Input: part model. Units: mm. Frame: model coordinates. Face numbers are marked on the shaded views. A direction names the side the tool comes from. Round coordinates to 2 decimals unless told otherwise and drop trailing zeros. Loops run counter-clockwise (first coordinate to the right, second up) from the corner with the lowest first, then second, coordinate; pieces in that order, holes last.
(1) First-contact query: pin 1 Ø12 at (x, y) = (-6, 8.5) entering from -Z; pin 2 Ø1.6 at (x, z) = (22.76, -15.21) entering from -Y; pin 3 Ø6 at (x, y) = (13.5, 15) entering from -Z. Flat tips, straight axial feed; report the tip coordinate or a pass-through.
(2) Access query for the marked faces 1 and 2. Directions: +Z, -Z, +X, -X, +Y, -Y. A direction counts if a zero-diameter tool reaches every point of the face in a straight line with its end or side. Return the directions, or none.
(3) Draft query along Z for the marked faces 3, 4 and 5. Return one class per face: released by +Z, released by -Z, zero draft, split by the parting line, or undercut.
(4) Cut plane D-D, the plane x = 8. Output: boundary loops of the cut face in (y, z), and give its area (3 significant figures).
(5) Cut plane B-B, the plane x = 0. Output: boundary loops of the cut face in (y, z).
(6) Cut plane A-A, the plane z = 0. Output: boundary loops of the cut face in (x, y), and give its area (3 significant figures).
(7) Cut plane C-C, the plane y = 30.5. Output: boundary loops of the cut face in (x, z).
(8) Line query: line 1 (Y direction, x = -7, z = -26.5); line 2 (X direction, y = 30.5, z = -1.5); line 3 (X direction, y = 24, z = -11). Output: solid intervals per line, ascending.
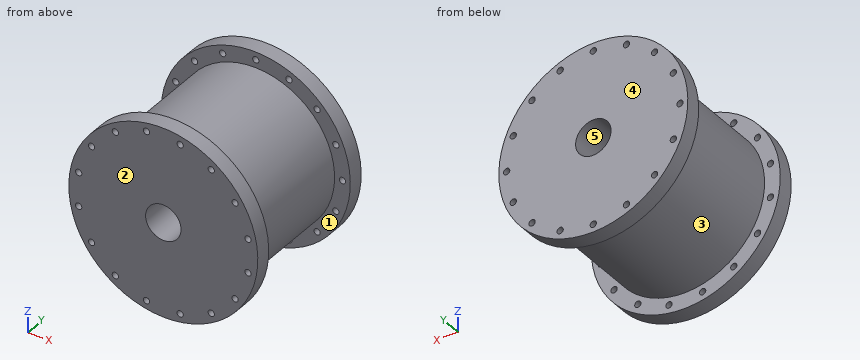
from build123d import *

# Parameters (mm, degrees)
SKETCH4_R          = 5.621513677
CUT_EXTRUDE1_DEPTH = 64.627776498
SKETCH5_R          = 1
CUT_EXTRUDE2_DEPTH = 60.991308336
CIRPATTERN2_COUNT  = 16
CUT_EXTRUDE3_REACH = 65.628
SKETCH7_R          = 1
CIRPATTERN3_COUNT  = 16


with BuildPart() as part:
    # Sketch3 → Revolve1 (revolve)
    with BuildSketch(Plane(origin=(0, 0, 0), x_dir=(0, 0, -1), z_dir=(1, 0, 0))):
        Polygon((29.972, 0), (0, 0), (0, 47.453686622), (29.972, 47.453686622), (29.972, 42.453686622), (24.993307857, 42.453686622), (24.993307857, 5), (29.972, 5), align=None)
    revolve(axis=Axis((0, 47.453686622, 0), (0, 1, 0)))

    # Sketch4 → Cut-Extrude1 (cut, through all)
    with BuildSketch(Plane(origin=(0, 47.453686622, 0), x_dir=(1, 0, 0), z_dir=(0, 1, 0))):
        with Locations(Location((0, 0, 0), (0, 0, 270))):
            Circle(SKETCH4_R)
    extrude(amount=-CUT_EXTRUDE1_DEPTH, mode=Mode.SUBTRACT)

    # Sketch5 → Cut-Extrude2 (cut, through all)
    with BuildSketch(Plane.XZ.offset(-42.453686622)):
        with Locations(Location((0, 27.482653928, 0), (0, 0, 270))):
            Circle(SKETCH5_R)
    cut_extrude2 = extrude(amount=-CUT_EXTRUDE2_DEPTH, mode=Mode.SUBTRACT)

    # CirPattern2: Cut-Extrude2 ×16 about axis
    cirpattern2_axis = Axis((0, 0, 0), (0, 1, 0))
    for i in range(1, CIRPATTERN2_COUNT):
        add(cut_extrude2.rotate(cirpattern2_axis, i * 360 / CIRPATTERN2_COUNT), mode=Mode.SUBTRACT)

    # Sketch7 → Cut-Extrude3 (cut, up to next)
    with BuildSketch(Plane.XZ, mode=Mode.PRIVATE) as cut_extrude3_sk1:
        with Locations(Location((-5.341086171, 26.85145344, 0), (0, 0, 270))):
            Circle(SKETCH7_R)
    cut_extrude3_tool1 = extrude(cut_extrude3_sk1.sketch, amount=-CUT_EXTRUDE3_REACH, mode=Mode.PRIVATE) & part.part
    cut_extrude3 = cut_extrude3_tool1.solids().sort_by_distance((-5.341086, 0, 26.851453))[0]
    add(cut_extrude3, mode=Mode.SUBTRACT)

    # CirPattern3: Cut-Extrude3 ×16 about axis
    cirpattern3_axis = Axis((0, 0, 0), (0, 1, 0))
    for i in range(1, CIRPATTERN3_COUNT):
        add(cut_extrude3.rotate(cirpattern3_axis, i * 360 / CIRPATTERN3_COUNT), mode=Mode.SUBTRACT)


solid = part.part
Reported:
1. pin 1: stops at z = -29.95
1. pin 2: stops at y = 42.45
1. pin 3: stops at z = -22.68
2. face 1: none
2. face 2: +Z, -Z, +X, -X, -Y
3. face 3: split by the parting line
3. face 4: zero draft
3. face 5: undercut
4. outline: (0, -28.88) - (5, -28.88) - (5, -23.68) - (42.45, -23.68) - (42.45, -28.88) - (47.45, -28.88) - (47.45, 28.88) - (42.45, 28.88) - (42.45, 23.68) - (5, 23.68) - (5, 28.88) - (0, 28.88) - close
4. area: 2,350 mm2
5. outline: (0, -29.97) - (5, -29.97) - (5, -24.99) - (42.45, -24.99) - (42.45, -26.48) - (47.45, -26.48) - (47.45, -5.62) - (0, -5.62) - close; (0, 5.62) - (47.45, 5.62) - (47.45, 26.48) - (42.45, 26.48) - (42.45, 24.99) - (5, 24.99) - (5, 29.97) - (0, 29.97) - close; (42.45, -29.97) - (47.45, -29.97) - (47.45, -28.48) - (42.45, -28.48) - close; (42.45, 28.48) - (47.45, 28.48) - (47.45, 29.97) - (42.45, 29.97) - close
6. outline: (-29.97, 0) - (-5.62, 0) - (-5.62, 47.45) - (-26.48, 47.45) - (-26.48, 42.45) - (-24.99, 42.45) - (-24.99, 5) - (-29.97, 5) - close; (-29.97, 42.45) - (-28.48, 42.45) - (-28.48, 47.45) - (-29.97, 47.45) - close; (5.62, 0) - (29.97, 0) - (29.97, 5) - (24.99, 5) - (24.99, 42.45) - (26.48, 42.45) - (26.48, 47.45) - (5.62, 47.45) - close; (28.48, 42.45) - (29.97, 42.45) - (29.97, 47.45) - (28.48, 47.45) - close
6. area: 1,920 mm2
7. outline: circle Ø49.99 at (0, 0); hole circle Ø11.24 at (0, 0)
8. line 1: y = 0 to 5, 42.45 to 47.45
8. line 2: x = -24.95 to -5.42, 5.42 to 24.95
8. line 3: x = -22.44 to 22.44
